Read the model definition and answer for the solid it produces. Units are mm, in the model's axes. Give positions to 0.01 mm unless a question says otherwise; leave off trailing zeros. Order: outer loops, then holes, each group sorted by start corner. A loop starts at its lowest first (then second) coordinate and runs counter-clockwise, first axis right, second up. Notation, with made-up numbers: (7.25, 14) - (42.25, 14) arc R21 cw to (42.25, 32) - close; hole circle Ø10 at (30, 15.25). An arc over 180 degrees is marked (long way). Write each question's results on one line, items separated by ' | '. Start each with the question number.
Q1. A flat-ended cylindrical pin translates along its axis: P1, Ø4, axis at x = 438.15, y = 36.83, coming from the +Z side. Find the tip coordinate at first contact, or state that the pin passes through.
Q2. Find the intervals of material crossed by line 1 along X through (y, z) = (36.83, 0.6); line 2 along Y through (x, z) = (222.36, 0.6); line 3 along Y through (x, z) = (438.15, 0.5), in increasing order. Write a range as from..to.
Q3. Find section A-A on y = 11.5. Give the vertices of the cut face in (x, z).
Autodesk Inventor part; units mm, degrees
ref_plane "YZ Plane" through (0, 0, 0) normal (1, 0, 0) x (0, 1, 0)
ref_plane "XZ Plane" through (0, 0, 0) normal (0, 1, 0) x (-1, 0, 0)
ref_plane "XY Plane" through (0, 0, 0) normal (0, 0, 1) x (1, 0, 0)
sketch "Sketch1" plane through (0, 0, 0) normal (0, 0, 1) x (1, 0, 0)
  line L0 (444.5, 63.5) -> (0, 63.5)
  line L1 (444.5, 30.48) -> (487.6052, 30.48) construction
  line L2 (0, 63.5) -> (0, 19.05)
  line L3 (0, 19.05) -> (35.921, 19.05) construction
  line L4 (0, 19.05) -> (28.7368, 19.05) construction
  line L5 (444.5, 63.5) -> (444.5, 19.05)
  line L6 (444.5, 19.05) -> (425.45, 0)
  line L7 (0, 19.05) -> (19.05, 0)
  line L8 (0, 19.05) -> (26.9408, 19.05) construction
  line L9 (19.05, 0) -> (425.45, 0)
  point P0 (0, 0)
  dimension "d0" = 444.5
  dimension "d38" = 44.45
  dimension "d41" = 44.45
  dimension "d42" = 135
  dimension "d43" = 45
extrude "Extrusion1" add sketch "Sketch1" along normal blind 1.5875
sketch "Sketch2" plane through (0, 0, 1.5875) normal (0, 0, 1) x (1, 0, 0)
  line L0 (0.22, 63.5) -> (0.22, 50.8)
  line L1 (0.22, 50.8) -> (12.92, 63.5)
  line L2 (444.5, 63.5) -> (0, 63.5)
  line L3 (0, 63.5) -> (0, 30.48)
  line L4 (0, 63.5) -> (6.57, 57.15)
  line L5 (6.57, 57.15) -> (6.57, 49.53)
  line L6 (6.57, 57.15) -> (14.19, 57.15) construction
  line L7 (444.5, 30.48) -> (444.5, 63.5)
  line L8 (444.5, 63.5) -> (444.5, 50.8)
  line L9 (444.5, 50.8) -> (431.8, 63.5)
  line L10 (431.8, 63.5) -> (444.5, 63.5)
  line L11 (444.5, 63.5) -> (438.15, 57.15)
  line L12 (438.15, 57.15) -> (438.15, 49.53)
  line L13 (438.15, 49.53) -> (6.57, 49.53)
  line L14 (20.32, 0) -> (414.02, 0)
  line L15 (429.26, 15.24) -> (444.5, 0)
  line L16 (425.45, 0) -> (444.5, 19.05)
  line L17 (434.975, 9.525) -> (419.7086, -5.7414)
  line L18 (438.15, 49.53) -> (438.15, 24.13)
  line L19 (6.57, 49.53) -> (6.57, 24.13)
  line L20 (6.57, 49.53) -> (31.97, 49.53) construction
  line L21 (222.36, 49.53) -> (222.36, 36.83)
  point P0 (0, 0)
  point P1 (0, 30.48)
  point P2 (30.48, 0)
  point P3 (25.4, 0)
  point P4 (415.2184, 20.3013)
  point P5 (6.57, 36.83)
  point P6 (438.15, 36.83)
  dimension "d9" = 12.7
  dimension "d10" = 45
  dimension "d20" = 7.62
  dimension "d21" = 90
  dimension "d22" = 12.7
  dimension "d23" = 45
  dimension "d24" = 7.62
  dimension "d44" = 21.59
  dimension "d48" = 25.4
  dimension "d49" = 25.4
  dimension "d50" = 90
hole "Hole2" at (6.57, 36.83, 1.5875) at (222.36, 36.83, 1.5875) at (438.15, 36.83, 1.5875) direction (0, 0, -1) diameter 4.7625 end through all
properties part number "sideskirt"
Working result:
1) P1: through
2) line 1: 0..4.19, 8.95..219.98, 224.74..435.77, 440.53..444.5 | line 2: 0..34.45, 39.21..63.5 | line 3: 12.7..34.45, 39.21..63.5
3) outline: (7.55, 0) - (436.95, 0) - (436.95, 1.59) - (7.55, 1.59) - close
